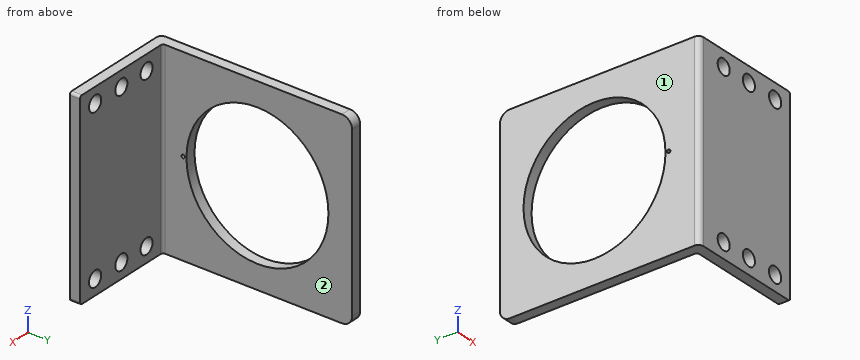
```python
from build123d import *

# Parameters (mm, degrees)
BOSS_EXTRUDE1_DEPTH = 37
SKETCH2_R           = 13.860055969
SKETCH2_R_2         = 0.332739378
CUT_EXTRUDE1_DEPTH  = 10
SKETCH3_R           = 1.513801081
SKETCH3_R_2         = 1.495226131
CUT_EXTRUDE2_DEPTH  = 10
FILLET1_R           = 2
FILLET2_R           = 0.5
FILLET3_R           = 0.5


with BuildPart() as part:
    # Sketch1 → Boss-Extrude1 (new body)
    with BuildSketch(Plane.XY):
        with BuildLine():
            Line((0, 0), (0, 37))
            Line((0, 37), (-2, 37))
            Line((-2, 37), (-2, -1))
            ThreePointArc((-2, -1), (-1.707106781, -1.707106781), (-1, -2))
            Line((-1, -2), (20.5, -2))
            Line((20.5, -2), (20.5, 0))
            Line((20.5, 0), (0, 0))
        make_face()
    extrude(amount=BOSS_EXTRUDE1_DEPTH)

    # Sketch2 → Cut-Extrude1 (cut)
    with BuildSketch(Plane(origin=(0, 0, 0), x_dir=(0, 0, -1), z_dir=(1, 0, 0))):
        with Locations((-18.5, 18.5)):
            Circle(SKETCH2_R)
        with Locations((-18.5, 4)):
            Circle(SKETCH2_R_2)
    extrude(amount=-CUT_EXTRUDE1_DEPTH, mode=Mode.SUBTRACT)

    # Sketch3 → Cut-Extrude2 (cut)
    with BuildSketch(Plane(origin=(0, 0, 0), x_dir=(1, 0, 0), z_dir=(0, 1, 0))):
        with Locations((16.75, -2.987028894)):
            Circle(SKETCH3_R)
        with Locations((10.25, -2.987028894)):
            Circle(SKETCH3_R_2)
        with Locations((4, -2.987028894)):
            Circle(SKETCH3_R_2)
        with Locations((16.75, -34.012971106)):
            Circle(SKETCH3_R)
        with Locations((10.25, -34.012971106)):
            Circle(SKETCH3_R_2)
        with Locations((4, -34.012971106)):
            Circle(SKETCH3_R_2)
    extrude(amount=-CUT_EXTRUDE2_DEPTH, mode=Mode.SUBTRACT)

    # Fillet1
    fillet1_edges = [part.edges().sort_by_distance(p)[0] for p in [
        (-1, 37, 37),
        (-1, 37, 0),
    ]]
    fillet(fillet1_edges, radius=FILLET1_R)

    # Fillet2
    fillet2_edges = [part.edges().sort_by_distance(p)[0] for p in [
        (0, 0, 18.5),
    ]]
    fillet(fillet2_edges, radius=FILLET2_R)

    # Fillet3
    fillet3_edges = [part.edges().sort_by_distance(p)[0] for p in [
        (20.5, -1, 37),
        (20.5, -1, 0),
    ]]
    fillet(fillet3_edges, radius=FILLET3_R)


solid = part.part
```
Model file for the job. Use its own axes, mm. Face numbers are marked on the shaded views. A direction names the side the tool comes from. Give positions to 0.01 mm unless a question says otherwise; leave off trailing zeros. Loops run counter-clockwise (first coordinate to the right, second up) from the corner with the lowest first, then second, coordinate; pieces in that order, holes last. Notation, with made-up numbers: (-28, 45) - (19, 45) arc R27 ccw to (19, 69) - close; hole circle Ø6 at (75.25, -25). An arc over 180 degrees is marked (long way). One line per item, written item: value. Start each with the question number.
1. Which spindle directions (+Z, -Z, +X, -X, +Y, -Y) get a long thin tool onto all of the face, cutting with end or side? Do the marked faces 1 and 2. Say none if no direction does.
2. Slice it at B-B (y = 6). List the corners of the cut face in (x, z), plus the area to 3 significant figures.
3. Probe L1, parallel to Z at x = 4, y = -1.55; L2, parallel to Y at x = -1.35, z = 18.5; L3, parallel to X at y = 1, z = 9. List the from-to ranges inside material, lowest first. Write a range as from..to.
4. Slice it at A-A (x = 4). List the corners of the cut face in (y, z).
5. Slice it at D-D (x = 16.75). List the corners of the cut face in (y, z), plus the area to 3 significant figures.
6. Pin check, flat tips, straight feed: pin 1 (2.5 mm diameter, centred on x = 16.75, z = 2.99, fed in from +Y); pin 2 (6 mm diameter, centred on y = 25, z = 8.5, fed in from -X); pin 3 (6 mm diameter, centred on y = 29.5, z = 27.5, fed in from +X); pin 4 (5 mm diameter, centred on x = 16.75, z = 34.01, fed in from +Y). Stop position of each tip, or through.
7. Slice it at C-C (z = 28.5). List the corners of the cut face in (x, y).
Solution:
1. face 1: +Z, -Z, -X, +Y, -Y
1. face 2: +Z, -Z, +X, +Y
2. outline: (-2, 0) - (0, 0) - (0, 12.51) - (-2, 12.51) - close; (-2, 24.49) - (0, 24.49) - (0, 37) - (-2, 37) - close
2. area: 50.0 mm^2
3. L1: z = 0..1.49, 4.48..32.52, 35.51..37
3. L2: y = -1.94..3.67, 4.33..4.64, 32.36..37
3. L3: x = -2..0
4. outline: (-2, 0) - (0, 0) - (0, 1.49) - (-2, 1.49) - close; (-2, 4.48) - (0, 4.48) - (0, 32.52) - (-2, 32.52) - close; (-2, 35.51) - (0, 35.51) - (0, 37) - (-2, 37) - close
5. outline: (-2, 0) - (0, 0) - (0, 1.47) - (-2, 1.47) - close; (-2, 4.5) - (0, 4.5) - (0, 32.5) - (-2, 32.5) - close; (-2, 35.53) - (0, 35.53) - (0, 37) - (-2, 37) - close
5. area: 61.9 mm^2
6. pin 1: passes through
6. pin 2: stops at x = -2
6. pin 3: stops at x = 0
6. pin 4: stops at y = 0
7. outline: (-2, -1) arc R1 ccw to (-1, -2) - (20.5, -2) - (20.5, 0) - (0.5, 0) arc R0.5 cw to (0, 0.5) - (0, 8.9) - (-2, 8.9) - close; (-2, 28.1) - (0, 28.1) - (0, 37) - (-2, 37) - close
